Can you work these out from the model? Positions are in its coordinate system, mm. A direction names the side the tool comes from. Round coordinates to 2 decimals unless told otherwise and drop trailing zeros. Order: outer loops, then holes, each group sorted by start corner. A loop starts at its lowest first (then second) coordinate and runs counter-clockwise, first axis right, second up.
Q1. If we section it at C-C (x = 75): Please give me the cut outline in (y, z).
Q2. If we section it at A-A (y = -5): Please give me the cut outline in (x, z), plus the area to 3 significant figures.
Q3. If we section it at D-D (y = 31): Please give me the cut outline in (x, z).
Q4. If I drill on line 1 (Z direction, x = 60, y = 28.75); line 2 (X direction, y = 30, z = 0); line 3 (Y direction, x = 0, z = 23), over which ranges is the centre line in solid material (lowest first)?
Q5. If we section it at B-B (z = 0): Count the separate pieces of the cut face and the enclosed holes in it, plus the area to 3 significant figures.
Q6. Will these pins go through, and if not, where does the flat tip stop? P1, Ø1.5, axis at y = 23.5, z = 23.5, coming from the -X side; P2, Ø0.9, axis at y = 35, z = 15.5, coming from the -X side; P3, Ø10, axis at x = -14.5, z = 15, coming from the -Y side; P4, Ø6.5, axis at x = 60, z = -36, coming from the -Y side.
Q7. We'd pull the mould along Z, two halves only. Please class faces 1 (the face through (63.905, 29.902, 35.133)), 2 (the face through (-19.71, -33.47, -12.7)), 3 (the face through (29.17, 22.53, 0.6)), 4 (the face through (92.27, 30.1, -24.44)): pulls with the +Z half, pulls with the -Z half, needs draft (parallel to the pull), parting line crosses it, or undercut.
Q8. For faces 5 (the face through (62.303, 38.479, -9.736)), 6 (the face through (11, 23, 43)), 7 (the face through (111.034, 29.902, -0.521)), which set-ups out of +Z, -Z, +X, -X, +Y, -Y let a thin tool reach every point of the face, with its end or its side?
Autodesk Inventor part; units mm, degrees
ref_plane "Work Plane1" through (0, 37, 43) normal (0, 1, 0) x (1, 0, 0)
ref_plane "Work Plane3" through (-31.8198, -31.8198, 0) normal (0.7071068, 0.7071068, 0) x (0, 0, 1)
ref_plane "YZ Plane" through (0, 0, 0) normal (1, 0, 0) x (0, 1, 0)
sketch "Sketch1" plane through (0, 0, 0) normal (0, 0, 1) x (1, 0, 0)
  circle A0 centre (0, 0) radius 25
  arc A1 (0, 34) -> (23.0434, 25) centre (0, 0) ccw
  line L0 (0, 34) -> (60, 34)
  line L1 (60, 34) -> (60, 25)
  line L2 (60, 25) -> (23.0434, 25)
  arc A2 (23.0434, 25) -> (0, 34) centre (0, 0) ccw construction
  dimension "d1" = 68
  dimension "d2" = 50
  dimension "d3" = 9
  dimension "d4" = 60
extrude "Extrusion1" add sketch "Sketch1" along normal mid plane 86
ref_plane "Work Plane1" through (0, 37, 43) normal (0, 1, 0) x (1, 0, 0)
sketch "Sketch2" plane through (0, 37, 43) normal (0, 1, 0) x (1, 0, 0)
  line L0 (60, 79) -> (115, 43) construction
  line L1 (115, 43) -> (60, 7) construction
  line L2 (60, 7) -> (60, 79) construction
  line L3 (60, 86) -> (60, 0)
  line L4 (119.3813, 49.6936) -> (64.3813, 85.6936)
  line L5 (52, 79) -> (52, 7)
  line L6 (64.3813, 0.3064) -> (119.3813, 36.3064)
  arc A0 (64.3813, 85.6936) -> (52, 79) centre (60, 79) ccw
  arc A1 (52, 7) -> (64.3813, 0.3064) centre (60, 7) ccw
  arc A2 (119.3813, 36.3064) -> (119.3813, 49.6936) centre (115, 43) ccw
  point P0 (0, 43)
  dimension "d8" = 55
  dimension "d9" = 72
  dimension "d10" = 8
  dimension "d11" = 8
extrude "Extrusion2" add sketch "Sketch2" against normal blind 14
sketch "Sketch3" plane through (0, 37, 43) normal (0, 1, 0) x (1, 0, 0)
  arc A0 (64.3813, 85.6936) -> (52, 79) centre (60, 79) ccw
  arc A1 (52, 7) -> (64.3813, 0.3064) centre (60, 7) ccw
  arc A2 (119.3813, 36.3064) -> (119.3813, 49.6936) centre (115, 43) ccw
  point P0 (0, 43)
hole "Hole1" at (60, 37, 36) at (60, 37, -36) at (115, 37, 0) direction (0, -1, 0) diameter 8 end through all
sketch "Sketch4" plane through (0, 37, 43) normal (0, 1, 0) x (1, 0, 0)
  circle A0 centre (115, 43) radius 4
  circle A1 centre (75, 43) radius 16
  point P0 (0, 43)
  dimension "d21" = 32
  dimension "d22" = 40
extrude "Extrusion3" add sketch "Sketch4" along normal blind 3 contours A1
sketch "Sketch5" plane through (75, 40, 0) normal (0, 1, 0) x (1, 0, 0)
  circle A0 centre (0, 0) radius 16
  point P0 (-75, 0)
hole "Hole2" at (75, 40, 0) direction (0, -1, 0) diameter 20 end through all
ref_plane "Work Plane3" through (-31.8198, -31.8198, 0) normal (0.7071068, 0.7071068, 0) x (0, 0, 1)
ref_plane "Work Plane2" through (0, 0, 0) normal (0.7071068, 0.7071068, 0) x (0, 0, 1)
sketch "Sketch6" plane through (-31.8198, -31.8198, 0) normal (0.7071068, 0.7071068, 0) x (0, 0, 1)
  circle A0 centre (0, 0) radius 16
  dimension "d34" = 32
extrude "Extrusion4" add sketch "Sketch6" along normal up to next
sketch "Sketch7" plane through (-31.8198, -31.8198, 0) normal (-0.7071068, -0.7071068, 0) x (-0.7071068, 0.7071068, 0)
  circle A0 centre (0, 0) radius 16
hole "Hole3" at (-31.8198, -31.8198, 0) direction (0.7071068, 0.7071068, 0) diameter 16.376 end up to surface
fillet "Fillet1" radius 5 1 edges at (23.0434, 25, 0)
properties part number "Part033.Pivoting connection" material "Steel, Carbon"
Solution:
1. outline: (23, -35.74) - (37, -35.74) - (37, -16) - (40, -16) - (40, -10) - (23, -10) - close; (23, 10) - (40, 10) - (40, 16) - (37, 16) - (37, 35.74) - (23, 35.74) - close
2. outline: (-33.63, -43) - (-24.49, -43) - (-24.49, 43) - (-33.63, 43) - close; (24.49, -43) - (33.63, -43) - (33.63, 43) - (24.49, 43) - close
2. area: 1,570 mm2
3. outline: (-13.96, -43) - (56.13, -43) arc R8 ccw to (64.38, -42.69) - (119.38, -6.69) arc R8 ccw to (119.38, 6.69) - (64.38, 42.69) arc R8 ccw to (56.13, 43) - (-13.96, 43) - close; hole circle Ø8 at (60, -36); hole circle Ø8 at (60, 36); hole circle Ø20 at (75, 0); hole circle Ø8 at (115, 0)
4. line 1: z = -44 to -40, -32 to 32, 40 to 44
4. line 2: x = -16 to 65, 85 to 111, 119 to 123
4. line 3: y = -34 to -25, 25 to 34
5. separate pieces: 3
5. enclosed holes: 0
5. area: 2,710 mm2
6. P1: stops at x = -25.27
6. P2: stops at x = 52
6. P3: stops at y = -33.93
6. P4: passes through
7. face 1: undercut
7. face 2: parting line crosses it
7. face 3: needs draft
7. face 4: pulls with the -Z half
8. face 5: +Y
8. face 6: +Z, -X, +Y, -Y
8. face 7: +Y, -Y
